Autodesk Inventor part; units mm, degrees
ref_plane "YZ Plane" through (0, 0, 0) normal (1, 0, 0) x (0, 1, 0)
ref_plane "XZ Plane" through (0, 0, 0) normal (0, 1, 0) x (-1, 0, 0)
ref_plane "XY Plane" through (0, 0, 0) normal (0, 0, 1) x (1, 0, 0)
sketch "Sketch1" plane through (0, 0, 0) normal (0, 1, 0) x (-1, 0, 0)
  line L0 (12.5, 12.5) -> (-12.5, 12.5)
  line L1 (-12.5, 12.5) -> (-12.5, -12.5)
  line L2 (-12.5, -12.5) -> (12.5, -12.5)
  line L3 (12.5, -12.5) -> (12.5, 12.5)
  line L4 (12.5, 12.5) -> (-12.5, -12.5) construction
  line L5 (-12.5, 12.5) -> (12.5, -12.5) construction
  point P0 (0, 0)
  dimension "d0" = 25
  dimension "d1" = 25
extrude "Extrusion1" add sketch "Sketch1" along normal blind 10
sketch "Sketch2" plane through (-12.5, 0, 12.5) normal (0, 0, 1) x (1, 0, 0)
  line L0 (25, 0) -> (25, 10)
  line L1 (0, 10) -> (25, 10)
  point P0 (12.5, 0)
  point P1 (12.5, 5.936)
  dimension "d12" = 4.064
hole "Hole1" at (0, 5.936, 12.5) direction (0, 0, -1) diameter 5 depth 25 counterbore diameter 7 counterbore depth 20
sketch "Sketch4" plane through (-12.5, 0, 12.5) normal (0, 0, 1) x (1, 0, 0)
  line L0 (4.5617, 5.936) -> (20.0475, 5.936) construction
  line L1 (8.0617, 9.436) -> (16.5475, 9.436)
  line L2 (16.5475, 2.436) -> (8.0617, 2.436)
  arc A0 (8.0617, 9.436) -> (8.0617, 2.436) centre (8.0617, 5.936) ccw
  arc A1 (16.5475, 2.436) -> (16.5475, 9.436) centre (16.5475, 5.936) ccw
  point P0 (12.5, 0)
  point P1 (12.3046, 5.936)
extrude "Extrusion2" cut sketch "Sketch4" against normal blind 20
sketch "Sketch5" plane through (-4.4383, 9.436, -7.5) normal (0, 0, 1) x (1, 0, 0)
  line L0 (-2.0833, -3.5) -> (10.4225, -3.5) construction
  line L1 (0.4167, -1) -> (7.9225, -1)
  line L2 (7.9225, -6) -> (0.4167, -6)
  arc A0 (0.4167, -1) -> (0.4167, -6) centre (0.4167, -3.5) ccw
  arc A1 (7.9225, -6) -> (7.9225, -1) centre (7.9225, -3.5) ccw
  point P0 (4.4383, -9.436)
  point P1 (4.1696, -3.5)
extrude "Extrusion3" cut sketch "Sketch5" against normal blind 20
sketch "Sketch6" plane through (-12.5, 0, -12.5) normal (-1, 0, 0) x (0, 0, 1)
  line L0 (25, 10) -> (0, 10)
  line L1 (0, 0) -> (25, 0)
  line L2 (0, 10) -> (25, 10)
  line L3 (25, 10) -> (25, 0)
  line L4 (25, 0) -> (0, 0)
  line L5 (0, 0) -> (0, 10)
  point P0 (12.5, 0)
extrude "Extrusion4" add sketch "Sketch6" along normal blind 5
sketch "Sketch7" plane through (12.5, 0, 12.5) normal (1, 0, 0) x (0, 0, -1)
  line L0 (0, 10) -> (25, 10)
  line L1 (0, 0) -> (25, 0)
  line L2 (0, 10) -> (25, 10)
  line L3 (25, 10) -> (25, 0)
  line L4 (25, 0) -> (0, 0)
  line L5 (0, 0) -> (0, 10)
  point P0 (12.5, 0)
extrude "Extrusion5" add sketch "Sketch7" along normal blind 5
sketch "Sketch8" plane through (0, 10, 0) normal (0, 1, 0) x (1, 0, 0)
  line L0 (-17.5, 12.5) -> (17.5, 12.5)
  line L1 (-17.5, -12.5) -> (-17.5, 12.5)
  line L2 (17.5, 12.5) -> (17.5, -12.5)
  point P0 (0, 0)
  point P1 (10, -4.917)
  point P2 (-10, -4.917)
  dimension "d28" = 17.417
  dimension "d29" = 17.417
  dimension "d30" = 7.5
  dimension "d31" = 7.5
hole "Hole2" at (10, 10, 4.917) at (-10, 10, 4.917) direction (0, -1, 0) diameter 3.302 depth 12.3
properties part number "ResonantAdapter"
Work out the finished part from the listing and answer in its coordinate system (mm). A direction names the side the tool comes from. Round coordinates to 2 decimals unless told otherwise and drop trailing zeros. Order: outer loops, then holes, each group sorted by start corner. A loop starts at its lowest first (then second) coordinate and runs counter-clockwise, first axis right, second up.
Q1. A cutting plane is placed at C-C, the plane y = 6.75. Determine the outline of the cut face in (x, z), then the cut area to 3 significant figures.
Solution:
outline: (-17.5, -12.5) - (-6.39, -12.5) - (-6.39, -7.5) - (-7.84, -7.5) - (-7.84, 12.5) - (-17.5, 12.5) - close; (5.85, -12.5) - (17.5, -12.5) - (17.5, 12.5) - (7.45, 12.5) - (7.45, -7.5) - (5.85, -7.5) - close; hole circle Ø3.3 at (-10, 4.92); hole circle Ø3.3 at (10, 4.92)
area: 491 mm2
Q2. A cutting plane is placed at A-A, the plane x = 10. Determine the outline of the cut face in (y, z), then the cut area to 3 significant figures.
Solution:
outline: (0, -12.5) - (10, -12.5) - (10, 3.27) - (0, 3.27) - close; (0, 6.57) - (10, 6.57) - (10, 12.5) - (0, 12.5) - close
area: 217 mm2
Q3. Find the intervals of material crossed by line 1 along Z through (x, y) = (-10, 3.25); line 2 along Y through (x, z) = (6.5, -6); line 3 along Y through (x, z) = (-2.5, 3.5), in increasing order.
Solution:
line 1: z = -12.5 to 3.27, 6.57 to 12.5
line 2: y = 0 to 3.44, 8.43 to 10
line 3: y = 0 to 2.44, 9.44 to 10
Q4. A cutting plane is placed at D-D, the plane z = 4.5. Determine the outline of the cut face in (x, y), then the cut area to 3 significant figures.
Solution:
outline: (-17.5, 0) - (-11.6, 0) - (-11.6, 10) - (-17.5, 10) - close; (-8.4, 0) - (8.4, 0) - (8.4, 10) - (-8.4, 10) - close; (11.6, 0) - (17.5, 0) - (17.5, 10) - (11.6, 10) - close; hole (-4.44, 2.44) - (4.05, 2.44) arc R3.5 ccw to (4.05, 9.44) - (-4.44, 9.44) arc R3.5 ccw to start
area: 188 mm2
Q5. A cutting plane is placed at B-B, the plane z = -10. Determine the outline of the cut face in (x, y), then the cut area to 3 significant figures.
Solution:
outline: (-17.5, 0) - (17.5, 0) - (17.5, 10) - (-17.5, 10) - close; hole (-4.02, 3.44) - (3.48, 3.44) arc R2.5 ccw to (3.48, 8.44) - (-4.02, 8.44) arc R2.5 ccw to start
area: 293 mm2
Q6. The mould has two halves that part along Y. Classify faces 1 (the flat face through (-17.5, 5, 0)), 2 (the flat face through (0, 10, 0)), 3 (the flat face through (0, 3.436, -10)): pulls with the +Y half, pulls with the -Y half, needs draft (parallel to the pull), parting line crosses it, or undercut.
Solution:
face 1: needs draft
face 2: pulls with the +Y half
face 3: undercut
Q7. A tool of negligible diameter and unlimited length cuts with its end or side. For faces 4 (the flat face through (0, 2.436, 3)), 5 (the cylindrical face through (5.984, 5.881, -9.965)), 6 (the cylindrical face through (11.465, 4.93, 5.679)), from which of +Z, -Z, +X, -X, +Y, -Y can it reach the whole face along a straight path? Write none if from no direction.
Solution:
face 4: +Z
face 5: +Z, -Z
face 6: +Y, -Y
